Source: CAD feature listing. Evaluate the final solid. Frame: model axes, mm. Face numbers are marked on the shaded views. A direction names the side the tool comes from. Round coordinates to 2 decimals unless told otherwise and drop trailing zeros. Loops run counter-clockwise (first coordinate to the right, second up) from the corner with the lowest first, then second, coordinate; pieces in that order, holes last. Notation, with made-up numbers: (74, 77.25) -> (90, 77.25) arc R29 cw to (90, 114.25) -> close; hole circle Ø9 at (-17.75, 63). An arc over 180 degrees is marked (long way). Write item = value, one per line.
from build123d import *

# Parameters (mm, degrees)
F0_R     = 10.795
F1_DEPTH = 4
F3_DEPTH = 6
F4_R     = 2
F5_R     = 3.05
F6_DEPTH = 25
F8_DEPTH = 4
F9_DEPTH = 25


with BuildPart() as f1:
    # F0 (on Top) → F1 (new body)
    with BuildSketch(Plane.XY):
        Circle(F0_R)
    extrude(amount=F1_DEPTH)

    # F2 (on face) → F3 (join)
    with BuildSketch(Plane.XY.offset(4)):
        with BuildLine():
            ThreePointArc((10.7673628762, 0.7719596449), (9.4157239289, 3.0593541588), (9.164726046, 5.704368633))
            ThreePointArc((9.164726046, 5.704368633), (6.3451417985, 8.7333384543), (2.5931208628, 10.4789192759))
            ThreePointArc((2.5931208628, 10.4789192759), (0, 9.9002780251), (-2.5931208628, 10.4789192759))
            ThreePointArc((-2.5931208628, 10.4789192759), (-6.3451417985, 8.7333384543), (-9.164726046, 5.704368633))
            ThreePointArc((-9.164726046, 5.704368633), (-9.129079829, 5.3250630068), (-9.1171822858, 4.94427191))
            ThreePointArc((-9.1171822858, 4.94427191), (-9.5447100851, 2.7008768479), (-10.7673628762, 0.7719596449))
            ThreePointArc((-10.7673628762, 0.7719596449), (-10.2666550934, -3.3358384543), (-8.2572330568, -6.9534255763))
            ThreePointArc((-8.2572330568, -6.9534255763), (-5.8192374168, -8.0094931714), (-4.0614753639, -10.0018219774))
            ThreePointArc((-4.0614753639, -10.0018219774), (0, -10.795), (4.0614753639, -10.0018219774))
            ThreePointArc((4.0614753639, -10.0018219774), (5.8192374168, -8.0094931714), (8.2572330568, -6.9534255763))
            ThreePointArc((8.2572330568, -6.9534255763), (10.1407311336, -3.7010264895), (10.795, 0))
            ThreePointArc((10.795, 0), (10.7880885065, 0.3862271041), (10.7673628762, 0.7719596449))
        make_face()
        with BuildLine():
            ThreePointArc((9.164726046, 5.704368633), (10.1650587649, 8.3626728896), (12.2607475986, 10.2797893132))
            ThreePointArc((12.2607475986, 10.2797893132), (9.4045640367, 12.94427191), (5.9878812408, 14.8372934947))
            ThreePointArc((5.9878812408, 14.8372934947), (4.8121986381, 12.2517534182), (2.5931208628, 10.4789192759))
            ThreePointArc((2.5931208628, 10.4789192759), (6.3451417985, 8.7333384543), (9.164726046, 5.704368633))
        make_face()
        with BuildLine():
            ThreePointArc((-2.5931208628, 10.4789192759), (-4.8121986381, 12.2517534182), (-5.9878812408, 14.8372934947))
            ThreePointArc((-5.9878812408, 14.8372934947), (-9.4045640367, 12.94427191), (-12.2607475986, 10.2797893132))
            ThreePointArc((-12.2607475986, 10.2797893132), (-10.1650587649, 8.3626728896), (-9.164726046, 5.704368633))
            ThreePointArc((-9.164726046, 5.704368633), (-6.3451417985, 8.7333384543), (-2.5931208628, 10.4789192759))
        make_face()
        with BuildLine():
            ThreePointArc((-10.7673628762, 0.7719596449), (-13.1391610839, -0.7906728554), (-15.961461726, -1.1098376324))
            ThreePointArc((-15.961461726, -1.1098376324), (-15.2169042607, -4.94427191), (-13.5654399842, -8.4840343019))
            ThreePointArc((-13.5654399842, -8.4840343019), (-11.0945504525, -7.0833373356), (-8.2572330568, -6.9534255763))
            ThreePointArc((-8.2572330568, -6.9534255763), (-10.2666550934, -3.3358384543), (-10.7673628762, 0.7719596449))
        make_face()
        with BuildLine():
            ThreePointArc((-3.876844616, -15.5232108735), (0, -16), (3.876844616, -15.5232108735))
            ThreePointArc((3.876844616, -15.5232108735), (3.3082494954, -12.7404161168), (4.0614753639, -10.0018219774))
            ThreePointArc((4.0614753639, -10.0018219774), (0, -10.795), (-4.0614753639, -10.0018219774))
            ThreePointArc((-4.0614753639, -10.0018219774), (-3.4970280206, -11.4251845557), (-3.3048420618, -12.94427191))
            ThreePointArc((-3.3048420618, -12.94427191), (-3.4495594274, -14.2650778287), (-3.876844616, -15.5232108735))
        make_face()
        with BuildLine():
            ThreePointArc((13.5654399842, -8.4840343019), (15.2169042607, -4.94427191), (15.961461726, -1.1098376324))
            ThreePointArc((15.961461726, -1.1098376324), (13.1391610839, -0.7906728554), (10.7673628762, 0.7719596449))
            ThreePointArc((10.7673628762, 0.7719596449), (10.7880885065, 0.3862271041), (10.795, 0))
            ThreePointArc((10.795, 0), (10.1407311336, -3.7010264895), (8.2572330568, -6.9534255763))
            ThreePointArc((8.2572330568, -6.9534255763), (11.0945504525, -7.0833373356), (13.5654399842, -8.4840343019))
        make_face()
    extrude(amount=F3_DEPTH)

    # F4
    f4_edges = [f1.edges().sort_by_distance(p)[0] for p in [
        (-5.987881, 14.837293, 7),
        (-12.260748, 10.279789, 7),
        (-15.961462, -1.109838, 7),
        (-13.56544, -8.484034, 7),
        (-3.876845, -15.523211, 7),
        (3.876845, -15.523211, 7),
        (13.56544, -8.484034, 7),
        (15.961462, -1.109838, 7),
        (12.260748, 10.279789, 7),
        (5.987881, 14.837293, 7),
    ]]
    fillet(f4_edges, radius=F4_R)

    # F5 (on face) → F6 (cut)
    with BuildSketch(Plane.XY.offset(10)):
        Circle(F5_R)
    extrude(amount=-F6_DEPTH, mode=Mode.SUBTRACT)

    # F7 (on face) → F8 (cut)
    with BuildSketch(Plane.XY.offset(10)):
        Polygon((2.8867513459, -5), (5.7735026919, 0), (2.8867513459, 5), (-2.8867513459, 5), (-5.7735026919, 0), (-2.8867513459, -5), align=None)
    extrude(amount=-F8_DEPTH, mode=Mode.SUBTRACT)

    # F2 (on face) → F9 (cut)
    with BuildSketch(Plane.XY.offset(4)):
        with BuildLine():
            ThreePointArc((-9.1171822858, 4.94427191), (-9.129079829, 5.3250630068), (-9.164726046, 5.704368633))
            ThreePointArc((-9.164726046, 5.704368633), (-10.2666550934, 3.3358384543), (-10.7673628762, 0.7719596449))
            ThreePointArc((-10.7673628762, 0.7719596449), (-9.5447100851, 2.7008768479), (-9.1171822858, 4.94427191))
        make_face()
        with BuildLine():
            ThreePointArc((-2.5931208628, 10.4789192759), (0, 9.9002780251), (2.5931208628, 10.4789192759))
            ThreePointArc((2.5931208628, 10.4789192759), (0, 10.795), (-2.5931208628, 10.4789192759))
        make_face()
        with BuildLine():
            ThreePointArc((10.7673628762, 0.7719596449), (10.2666550934, 3.3358384543), (9.164726046, 5.704368633))
            ThreePointArc((9.164726046, 5.704368633), (9.4157239289, 3.0593541588), (10.7673628762, 0.7719596449))
        make_face()
        with BuildLine():
            ThreePointArc((4.0614753639, -10.0018219774), (6.3451417985, -8.7333384543), (8.2572330568, -6.9534255763))
            ThreePointArc((8.2572330568, -6.9534255763), (5.8192374168, -8.0094931714), (4.0614753639, -10.0018219774))
        make_face()
        with BuildLine():
            ThreePointArc((-8.2572330568, -6.9534255763), (-6.3451417985, -8.7333384543), (-4.0614753639, -10.0018219774))
            ThreePointArc((-4.0614753639, -10.0018219774), (-5.8192374168, -8.0094931714), (-8.2572330568, -6.9534255763))
        make_face()
    extrude(amount=-F9_DEPTH, mode=Mode.SUBTRACT)


solid = f1.part
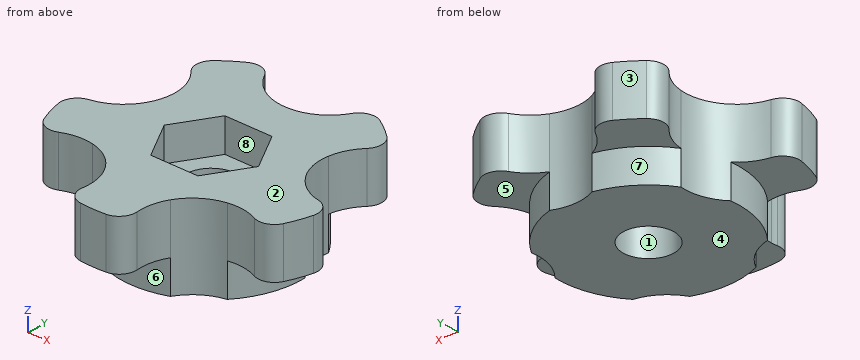
1. Section query B-B (y = 4.5). Return the cut outline in (x, z), then the cut area to 3 significant figures.
Evaluation:
outline = (-9.13, 0) -> (9.13, 0) -> (9.13, 10) -> (3.18, 10) -> (3.18, 6) -> (-3.18, 6) -> (-3.18, 10) -> (-9.13, 10) -> close
area = 157 mm²
2. Line query: probe 1 along Y at (x, z) = (0, 1.45) (3 decimals); probe 2 along Y at (x, z) = (0, 4.7); probe 3 along Z at (x, y) = (12, -3.5). Output: solid intervals per line, ascending. Write a range as from..to.
Evaluation:
probe_1 = -10.795..-3.05, 3.05..9.9
probe_2 = -16..-3.05, 3.05..9.9
probe_3 = 4..10
3. Set-up query: the marked faces 4, 5, 6, 7 and 8. Return all of +Z, -Z, +X, -X, +Y, -Y with unobstructed straight access to the full face (end or side cutting, diameter ignored); none if empty.
Evaluation:
face_4 = -Z, +X, -X, +Y, -Y
face_5 = -Z, +X, +Y
face_6 = -Z, -Y
face_7 = -Z, -X, +Y
face_8 = +Z
4. Section query C-C (z = 3.5). Return the cut outline in (x, y) (3 decimals), then the cut area to 3 significant figures.
Evaluation:
outline = (-10.767, 0.772) arc R10.795 ccw to (-8.257, -6.953) arc R6.1 cw to (-4.061, -10.002) arc R10.795 ccw to (4.061, -10.002) arc R6.1 cw to (8.257, -6.953) arc R10.795 ccw to (10.767, 0.772) arc R6.1 cw to (9.165, 5.704) arc R10.795 ccw to (2.593, 10.479) arc R6.1 cw to (-2.593, 10.479) arc R10.795 ccw to (-9.165, 5.704) arc R6.1 cw to start; hole circle Ø6.1 at (0, 0)
area = 321 mm²
5. Mould query, pull axis Y, two halves, no side actions, for the marked faces 1, 2 and 3. Classes: released by +Y, released by -Y, zero draft, split by the parting line, or undercut.
Evaluation:
face_1 = undercut
face_2 = zero draft
face_3 = released by +Y
6. Section query A-A (x = 0). Return the cut outline in (y, z) (3 decimals).
Evaluation:
outline = (-16, 4) -> (-10.795, 4) -> (-10.795, 0) -> (-3.05, 0) -> (-3.05, 6) -> (-5, 6) -> (-5, 10) -> (-16, 10) -> close; (3.05, 0) -> (9.9, 0) -> (9.9, 10) -> (5, 10) -> (5, 6) -> (3.05, 6) -> close
7. Contact query for flat-ended pins moving along their axis: pin 1 Ø1 at (y, z) = (-6.5, 4.5) entering from -X; pin 2 Ø3.5 at (x, y) = (0, 0) entering from +Z; pin 3 Ø3 at (x, y) = (1, -13) entering from -Z; pin 4 Ø1 at (x, z) = (8.5, 4.5) entering from -Y. Output: stop coordinate, or through.
Evaluation:
pin_1 = -14.83
pin_2 = through
pin_3 = 4
pin_4 = -7.01
